The listing builds one solid part. Answer for the finished solid, in the listing's coordinates (mm). Face numbers are marked on the shaded views. Give positions to 0.01 mm unless a question says otherwise; leave off trailing zeros. Write each loop counter-clockwise with the first axis right and the second up, starting at its lowest first coordinate (ties: lowest second). Pieces come first, ordered by that corner, then holes.
Autodesk Inventor part; units mm, degrees
ref_plane "MSC_PF1" through (0, 0, 0) normal (1, 0, 0) x (0, 1, 0)
ref_plane "MSC_PT1" through (0, 0, 0) normal (0, 0, -1) x (-1, 0, 0)
ref_plane "YZ Plane" through (0, 0, 0) normal (1, 0, 0) x (0, 1, 0)
sketch "Sketch1" plane through (0, 0, 0) normal (0, 1, 0) x (-1, 0, 0)
  point P0 (0, 0)
sketch "Sketch2" plane through (0, 0, 0) normal (0, 1, 0) x (-1, 0, 0)
  line L0 (-2, -40) -> (0, -40)
  line L1 (-2, -2.3) -> (-2, -40)
  line L2 (-4, -0.3) -> (-2, -2.3)
  line L3 (-4, 0) -> (-4, -0.3)
  line L4 (0, 0) -> (-4, 0)
  line L5 (0, -40) -> (0, 0)
  line L6 (0, -40) -> (0, 0)
  line L7 (0, -48) -> (0, 8)
  line L8 (0.8, 0) -> (-4.8, 0)
  dimension "d3" = 4
  dimension "d5" = 2
  dimension "d7" = 40
  dimension "ParC" = 0.3
  dimension "d22" = 0
  dimension "d23" = 0
  dimension "d43" = 45
revolve "Revolution1" add sketch "Sketch2" angle 360 about axis through (0, 0, -40) along (0, 0, -1)
sketch "Sketch3" plane through (0, 0, 0) normal (0, 0, 1) x (1, 0, 0)
  line L0 (-1.25, 0.7217) -> (-1.25, -0.7217)
  line L1 (0, 1.4434) -> (-1.25, 0.7217)
  line L2 (1.25, 0.7217) -> (0, 1.4434)
  line L3 (1.25, -0.7217) -> (1.25, 0.7217)
  line L4 (0, -1.4434) -> (1.25, -0.7217)
  line L5 (-1.25, -0.7217) -> (0, -1.4434)
  circle A0 centre (0, 0) radius 1.25 construction
  circle A1 centre (0, 0) radius 2 construction
  dimension "d11" = 2.5
  dimension "d13" = 120
  dimension "d15" = 120
extrude "Extrusion1" cut sketch "Sketch3" against normal blind 1.8
fillet "Fillet1" radius 0.2 1 edges at (-2, 0, -2.3)
chamfer "Chamfer1" distance 0.35 angle 45 1 edges at (-2, 0, -40) measured on face at (-0.9288, -1.7713, -27.4609)
thread "Thread1"
ref_plane "MSC_PF1" through (0, 0, 0) normal (1, 0, 0) x (0, 1, 0)
ref_plane "MSC_PT1" through (0, 0, 0) normal (0, 0, -1) x (-1, 0, 0)
equation "\"d3\" = 0.5 * dk"
equation "\"d5\" = 0.5 * NND"
equation "\"d7\" = NLG"
equation "\"d43\" = 0.5 * ang"
equation "\"d18\" = r"
equation "\"d19\" = 0.5 * PTC"
equation "\"d39\" = 0.5 * PTC"
equation "\"d11\" = ParS"
equation "\"d16\" = ParT"
equation "\"NND\" = 4"
equation "\"PTC\" = 0.7"
equation "\"dk\" = 8"
equation "\"ParK\" = 2.3"
equation "\"ParS\" = 2.5"
equation "\"ParT\" = 1.8"
equation "\"r\" = 0.2"
equation "\"NLG\" = 40"
equation "\"ang\" = 90deg"
equation "\"THREADDIA\" = NND"
properties part number "DIN 7991 - M4x40" material "Steel, Mild"
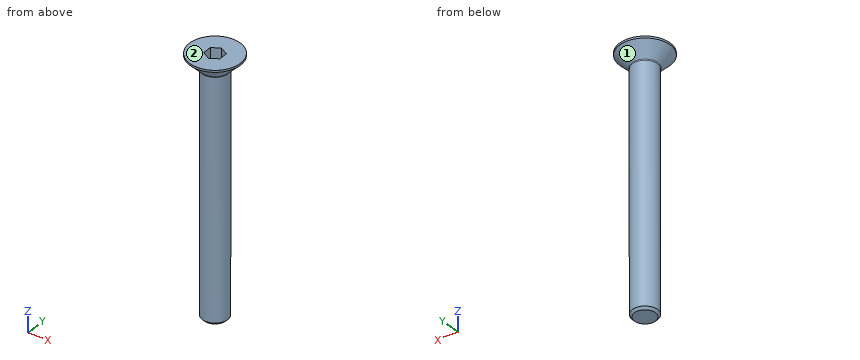
Item 1: A cutting plane is placed at A-A, the plane z = -34.5. Give the vertices of the cut face in (x, y), plus the area to 3 significant figures.
Conclusion:
outline: circle Ø4 at (0, 0)
area: 12.6 mm2
Item 2: Consider probe 1 along Z at (x, y) = (0.5, -0.25); probe 2 along Z at (x, y) = (-0.5, -3); probe 3 along Y at (x, z) = (-2.5, -1.5). Determine where each line is inside the solid, lowest interval first.
Conclusion:
probe 1: z = -40 to -1.8
probe 2: z = -1.26 to 0
probe 3: y = -1.26 to 1.26
Item 3: Determine the mould class of the marked faces 1 and 2 for opening direction X: pulls with the +X half, pulls with the -X half, needs draft (parallel to the pull), parting line crosses it, or undercut.
Conclusion:
face 1: parting line crosses it
face 2: needs draft
Item 4: Each of these flat-tipped pins is pushed along its axis until it touches: P1, Ø2, axis at x = -0.5, y = -0.5, coming from the +Z side; P2, Ø1.5, axis at y = 2, z = -11, coming from the +X side; P3, Ø1.5, axis at x = 0, z = -24, coming from the +Y side. Where does it stop, or does it pass through?
Conclusion:
P1: stops at z = 0
P2: stops at x = 1.56
P3: stops at y = 2
